```python
from build123d import *

# Parameters (mm, degrees)
BOSS_EXTRU_1_DEPTH = 10
CONG_1_R           = 2


with BuildPart() as part:
    # Esquisse1 → Boss.-Extru.1 (new body)
    with BuildSketch(Plane.XY):
        with BuildLine():
            Line((0, 0), (95.5, 0))
            Line((95.5, 0), (95.5, 5))
            Line((95.5, 5), (80.339854507, 22.251465861))
            Line((80.339854507, 22.251465861), (75.339854507, 22.251465861))
            Line((75.339854507, 22.251465861), (75.485610115, 5.549527541))
            Line((75.485610115, 5.549527541), (65, 5))
            Line((65, 5), (63.338872772, 22.251465861))
            Line((63.338872772, 22.251465861), (58.36189178, 21.772237099))
            ThreePointArc((58.36189178, 21.772237099), (32.967836132, 9.291799024), (5, 5))
            Line((5, 5), (0, 5))
            Line((0, 5), (0, 0))
        make_face()
    extrude(amount=BOSS_EXTRU_1_DEPTH)

    # Congé1
    cong_1_edges = [part.edges().sort_by_distance(p)[0] for p in [
        (0, 5, 5),
        (58.36189178, 21.772237099, 5),
        (63.338872772, 22.251465861, 5),
        (75.339854507, 22.251465861, 5),
        (80.339854507, 22.251465861, 5),
        (95.5, 5, 5),
    ]]
    fillet(cong_1_edges, radius=CONG_1_R)


solid = part.part
```
The model under review builds one solid part; all positions refer to its coordinate system, in mm. A direction names the side the tool comes from. Coordinates: 2 decimals unless noted, no trailing zeros. Write each loop counter-clockwise with the first axis right and the second up, starting at its lowest first coordinate (ties: lowest second). Pieces come first, ordered by that corner, then holes. Notation, with made-up numbers: (86.25, 30.25) - (102.25, 30.25) arc R23 ccw to (102.25, 69.25) - close; hole circle Ø8 at (87.25, -21). An arc over 180 degrees is marked (long way). Answer in a Markdown table with one row per item. Add a question column.
Q1. Draft analysis for pull direction X (two halves, no side actions). For faces 3 (the face through (80.27, 22.07, 5.07)), 4 (the face through (33.098, 9.333, 4.93)), 5 (the face through (4, 5, 5)), 6 (the face through (62.829, 21.598, 5.07)), state which applies: +X half, -X half, draft (parallel to the pull), parting line (faces both ways), or undercut.
Q2. Consider section C-C on y = 18. Give the boundary of the cut face in (x, z).
Q3. To check wall thickness, follow line 1 along X through (y, z) = (11.75, 7.25); line 2 along X through (y, z) = (20.75, 9); line 3 along Y through (x, z) = (62.5, 3.5). State the ranges of each line that lie inside material, in increasing order. Write a range as from..to.
Q4. Consider section B-B on z = 1.75. Give the boundary of the cut face in (x, y), then the cut area to 3 significant figures.
Q5. Consider section D-D on x = 53.5. Give the boundary of the cut face in (y, z).
Q6. Consider section A-A on y = 10.5. Give the boundary of the cut face in (x, z), then the cut area to 3 significant figures.
Q7. For faces 1 (the face through (64.276, 12.524, 4.93)), 2 (the face through (47, 0, 5)), list the 3-axis set-ups (+Z, -Z, +X, -X, +Y, -Y) from which the entire face can be reached by the end or side of a thin tool; tool diameter is ignored.
Q8. Clearance check with flat-ended pins moving along their axes: pin 1 (3.5 mm diameter, centred on x = 3, z = 5.5, fed in from +Y); pin 2 (2 mm diameter, centred on y = 14.5, z = 6, fed in from -X). State where each tip first meets the part, or that it passes through.
Answers below:
| question | item | result |
|---|---|---|
| 1 | face 3 | +X half |
| 1 | face 4 | -X half |
| 1 | face 5 | draft |
| 1 | face 6 | undercut |
| 2 | outline | (52.5, 0) - (63.75, 0) - (63.75, 10) - (52.5, 10) - close; (75.38, 0) - (84.08, 0) - (84.08, 10) - (75.38, 10) - close |
| 3 | line 1 | 39.84..64.35, 75.43..89.57 |
| 3 | line 2 | 56.87..63.42, 75.42..81.66 |
| 3 | line 3 | 0..21.82 |
| 4 | outline | (0, 0) - (95.5, 0) - (95.5, 4.25) arc R2 ccw to (95, 5.57) - (80.94, 21.57) arc R2 ccw to (79.43, 22.25) - (77.36, 22.25) arc R2 ccw to (75.36, 20.23) - (75.49, 5.55) - (65, 5) - (63.53, 20.26) arc R2 ccw to (61.35, 22.06) - (58.88, 21.82) arc R2 ccw to (57.94, 21.48) arc R93.27 cw to (5, 5) - (2, 5) arc R2 ccw to (0, 3) - close |
| 4 | area | 1,080 mm² |
| 5 | outline | (0, 0) - (18.6, 0) - (18.6, 10) - (0, 10) - close |
| 6 | outline | (36.56, 0) - (64.47, 0) - (64.47, 10) - (36.56, 10) - close; (75.44, 0) - (90.67, 0) - (90.67, 10) - (75.44, 10) - close |
| 6 | area | 431 mm² |
| 7 | face 1 | +Z, -Z, +Y |
| 7 | face 2 | +Z, -Z, +X, -X, -Y |
| 8 | pin 1 | y = 5 |
| 8 | pin 2 | x = 43.9 |
